```python
from build123d import *

# Parameters (mm, degrees)
F1_DEPTH       = 15
F2_R           = 2
F4_DEPTH       = 4.5
F6_DEPTH       = 4.5
F7_R           = 2
F8_SIZE        = 1
F10_DEPTH      = 2
F10_DEPTH_BACK = 8
F12_DEPTH      = 5
F14_DEPTH      = 1
F15_R          = 10
F16_R          = 3
F17_R          = 2
F18_T1_DEPTH   = 27


# Not quite as in the source:
# - a fillet or chamfer that OpenCascade refuses, or shapes differently, is made with other operations: its cross-section is extruded or revolved along the edge and cut away or added


with BuildPart() as f1:
    # F0 (on Top) → F1 (new body)
    with BuildSketch(Plane.XY):
        Polygon((-8.0448907178, 7.5019819607), (0, 0), (15.0350819326, 5.4723222932), (25.8464898551, 56.3359975314), (19.5579639798, 92), (-3.4420360202, 92), (-8.030647511, 85.4467836457), (-6.4537553867, 81.7707244475), (-13.8947211419, 53.7415962301), (-16.7171564284, 43.1098579407), (-19.7961767409, 31.5115979887), (-9.299232277, 19.4362447051), align=None)
        with BuildLine():
            ThreePointArc((-13.8947211419, 53.7415962301), (-18.2055037731, 49.1954821635), (-16.7171564284, 43.1098579407))
            Line((-16.7171564284, 43.1098579407), (-13.8947211419, 53.7415962301))
        make_face()
    extrude(amount=F1_DEPTH)

    # F2
    f2_edges = [f1.edges().sort_by_distance(p)[0] for p in [
        (-3.442036, 92, 7.5),
        (19.557964, 92, 7.5),
        (-8.030648, 85.446784, 7.5),
        (-6.453755, 81.770724, 7.5),
        (25.84649, 56.335998, 7.5),
        (15.035082, 5.472322, 7.5),
        (-19.796177, 31.511598, 7.5),
        (-8.044891, 7.501982, 7.5),
        (0, 0, 7.5),
    ]]
    fillet(f2_edges, radius=F2_R)

    # F3 (on face) → F4 (cut)
    with BuildSketch(Plane.XY.offset(15)):
        with BuildLine():
            Line((-19.1004557272, 30.7112625143), (-9.299232277, 19.4362447051))
            Line((-9.299232277, 19.4362447051), (-9.9431083431, 25.5623162612))
            ThreePointArc((-9.9431083431, 25.5623162612), (-4.1654007718, 41.7730592838), (-4.2262892289, 58.9825446545))
            Line((-4.2262892289, 58.9825446545), (0.2837840411, 62.9397203012))
            Line((0.2837840411, 62.9397203012), (-1.9921549357, 80.795254507))
            Line((-1.9921549357, 80.795254507), (-6.7258938789, 82.4051351292))
            ThreePointArc((-6.7258938789, 82.4051351292), (-6.5692308005, 81.7622951194), (-6.6308801526, 81.103519015))
            Line((-6.6308801526, 81.103519015), (-13.8947211419, 53.7415962301))
            ThreePointArc((-13.8947211419, 53.7415962301), (-18.2055037731, 49.1954821635), (-16.7171564284, 43.1098579407))
            Line((-16.7171564284, 43.1098579407), (-19.5240798921, 32.5365506243))
            ThreePointArc((-19.5240798921, 32.5365506243), (-19.539255282, 31.5712259114), (-19.1004557272, 30.7112625143))
        make_face()
    extrude(amount=-F4_DEPTH, mode=Mode.SUBTRACT)

    # F5 (on face) → F6 (cut)
    with BuildSketch(Plane(origin=(0, 0, 0), x_dir=(1, 0, 0), z_dir=(0, 0, -1))):
        with BuildLine():
            ThreePointArc((-6.6308801526, -81.103519015), (-6.5692308005, -81.7622951194), (-6.7258938789, -82.4051351292))
            Line((-6.7258938789, -82.4051351292), (-2.0079532375, -80.7495276563))
            Line((-2.0079532375, -80.7495276563), (0.2709017201, -62.8943653752))
            Line((0.2709017201, -62.8943653752), (-4.2385252382, -58.9364532352))
            ThreePointArc((-4.2385252382, -58.9364532352), (-4.1797341848, -41.7514896804), (-9.9430388376, -25.5616549609))
            Line((-9.9430388376, -25.5616549609), (-9.299232277, -19.4362447051))
            Line((-9.299232277, -19.4362447051), (-19.1004557272, -30.7112625143))
            ThreePointArc((-19.1004557272, -30.7112625143), (-19.539255282, -31.5712259114), (-19.5240798921, -32.5365506243))
            Line((-19.5240798921, -32.5365506243), (-16.7171564284, -43.1098579407))
            ThreePointArc((-16.7171564284, -43.1098579407), (-18.2055037731, -49.1954821635), (-13.8947211419, -53.7415962301))
            Line((-13.8947211419, -53.7415962301), (-6.6308801526, -81.103519015))
        make_face()
    extrude(amount=-F6_DEPTH, mode=Mode.SUBTRACT)

    # F7
    f7_edges = [f1.edges().sort_by_distance(p)[0] for p in [
        (-9.943108, 25.562316, 12.75),
        (-9.943039, 25.561655, 2.25),
        (-4.226289, 58.982545, 12.75),
        (0.283784, 62.93972, 12.75),
        (-4.238525, 58.936453, 2.25),
        (0.270902, 62.894365, 2.25),
        (-1.992155, 80.795255, 12.75),
        (-2.007953, 80.749528, 2.25),
        (-6.725894, 82.405135, 7.5),
        (-6.725894, 82.405135, 2.25),
        (-6.725894, 82.405135, 12.75),
    ]]
    fillet(f7_edges, radius=F7_R)

    # F8
    f8_edges = [f1.edges().sort_by_distance(p)[0] for p in [
        (-7.334289, 83.82343, 15),
        (-6.597337, 82.544049, 15),
        (-7.743054, 85.417108, 15),
        (-4.528565, 81.657853, 15),
        (-5.715563, 88.753067, 15),
        (-2.269238, 80.568943, 15),
        (-3.324399, 91.774022, 15),
        (-0.842477, 71.775634, 15),
        (7.739431, 92, 15),
        (0.035819, 63.033597, 15),
        (19.16534, 91.532089, 15),
        (-1.952405, 60.977669, 15),
        (22.814181, 73.533074, 15),
        (-3.950317, 58.895605, 15),
        (25.809062, 56.336651, 15),
        (-4.205609, 41.541288, 15),
        (20.515619, 31.256223, 15),
        (-9.848308, 25.536603, 15),
        (14.818701, 5.66042, 15),
        (-8.999956, 16.588822, 15),
        (7.572505, 2.756166, 15),
        (-7.923879, 7.562316, 15),
        (0.068913, 0.338716, 15),
        (-4.197178, 3.913931, 15),
        (-7.332009, 83.818114, 0),
        (-6.599862, 82.540006, 0),
        (-7.743054, 85.417108, 0),
        (-4.534925, 81.636286, 0),
        (-5.715563, 88.753067, 0),
        (-2.280519, 80.529059, 0),
        (-3.324399, 91.774022, 0),
        (-0.857666, 71.736857, 0),
        (7.739431, 92, 0),
        (0.022922, 62.988201, 0),
        (19.16534, 91.532089, 0),
        (-1.965224, 60.931724, 0),
        (22.814181, 73.533074, 0),
        (-3.962878, 58.849592, 0),
        (25.809062, 56.336651, 0),
        (-4.219912, 41.519712, 0),
        (20.515619, 31.256223, 0),
        (-9.848432, 25.536019, 0),
        (14.818701, 5.66042, 0),
        (-8.999957, 16.588832, 0),
        (7.572505, 2.756166, 0),
        (-7.923879, 7.562316, 0),
        (0.068913, 0.338716, 0),
        (-4.197178, 3.913931, 0),
    ]]
    chamfer(f8_edges, length=F8_SIZE)

    # F9 (on face) → F10 (join, two sides)
    with BuildSketch(Plane.XY.offset(10.5)) as f10_sk:
        Polygon((-9.2121738851, 71.3801288833), (-11.82835392, 61.5253266909), (-8.928788932, 60.7555716127), (-7.6458638018, 65.5881799261), (-5.5294538555, 67.7143993266), align=None)
    extrude(amount=F10_DEPTH)
    extrude(f10_sk.sketch, amount=-F10_DEPTH_BACK)

    # F11 (on face) → F12 (join)
    with BuildSketch(Plane(origin=(0, 0, 0), x_dir=(1, 0, 0), z_dir=(0, 0, -1))):
        Polygon((5.5166269788, -69.1855618273), (14.7091602962, -76.8990131435), (15.3519479059, -76.1329687004), (6.1594145885, -68.4195173842), align=None)
    extrude(amount=F12_DEPTH)

    # F13 (on face) → F14 (join)
    with BuildSketch(Plane(origin=(0, 0, -5), x_dir=(1, 0, 0), z_dir=(0, 0, -1))):
        Polygon((6.1594145885, -68.4195173842), (15.3519479059, -76.1329687004), (18.3099562872, -59.3572695449), (9.9443103961, -20), (4.371628125, -21.1845101828), (8.5288556293, -61.3816455007), align=None)
        Polygon((14.7091602962, -76.8990131435), (15.3519479059, -76.1329687004), (6.1594145885, -68.4195173842), (5.5166269788, -69.1855618273), align=None)
    extrude(amount=-F14_DEPTH)

    # F15
    f15_edges = [f1.edges().sort_by_distance(p)[0] for p in [
        (18.309956, 59.35727, -4.5),
        (8.528856, 61.381646, -4.5),
    ]]
    fillet(f15_edges, radius=F15_R)

    # F16
    f16_edges = [f1.edges().sort_by_distance(p)[0] for p in [
        (4.371628, 21.18451, -4.5),
        (9.94431, 20, -4.5),
    ]]
    fillet(f16_edges, radius=F16_R)

    # F17
    f17_edges = [f1.edges().sort_by_distance(p)[0] for p in [
        (10.755681, 72.276243, -4),
    ]]
    fillet(f17_edges, radius=F17_R)

    # F18: fillet of radius 3 on 1 edges, made by hand

    # F18_s2 → F18_t1 (cut)
    with BuildSketch(Plane(origin=(31.5591951189, 26.4813089845, 0), x_dir=(0, 0, 1), z_dir=(0.7660444431, 0.6427876097, 0))):
        with BuildLine():
            ThreePointArc((-5, -46.4531957126), (-4.1213203436, -48.5745160562), (-2, -49.4531957126))
            Line((-2, -49.4531957126), (-5, -49.4531957126))
            Line((-5, -49.4531957126), (-5, -46.4531957126))
        make_face()
    extrude(amount=F18_T1_DEPTH, mode=Mode.SUBTRACT)


solid = f1.part
```
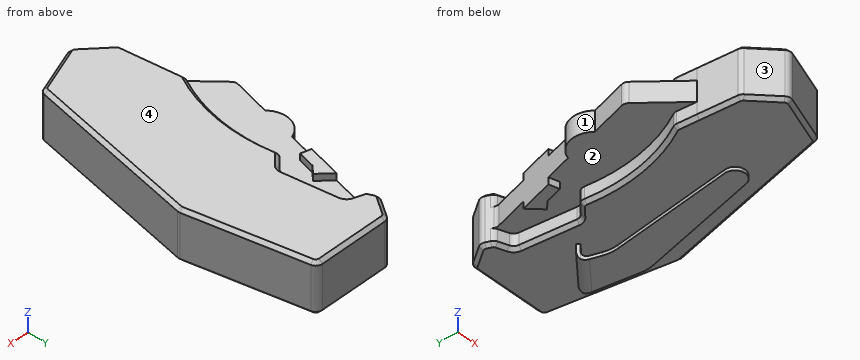
The model under review builds one solid part; all positions refer to its coordinate system, in mm. Face numbers are marked on the shaded views. Give positions to 0.01 mm unless a question says otherwise; leave off trailing zeros. Order: outer loops, then holes, each group sorted by start corner. A loop starts at its lowest first (then second) coordinate and runs counter-clockwise, first axis right, second up. Notation, with made-up numbers: (73.25, -15.5) - (84.25, -15.5) arc R28 ccw to (84.25, 14.5) - close; hole circle Ø2 at (-37.5, 5.25). An arc over 180 degrees is marked (long way). Use CSV: the item, a comma, the result in double quotes. Start each with the question number.
Q1. We need section B-B, the plane x = 21. Write out the cut boundary in (y, z), and give its area (3 significant figures).
Q2. The part is to be moulded in two halves that separate along Y. For the marked faces 1, 2, 3 and 4, say which applies: +Y half, -Y half, draft (parallel to the pull), parting line (faces both ways), or undercut.
Q3. To check wall thickness, follow line 1 along Z through (x, y) = (6.5, 33.5); line 2 along Z through (x, y) = (-8, 68); line 3 along Z through (x, y) = (-6, 84). State the ranges of each line that lie inside material, in increasing order. Write a range as [from, to].
Q4. Clearance check with flat-ended pins moving along their axes: pin 1 Ø1 at (y, z) = (33.5, 12) entering from +X; pin 2 Ø6 at (y, z) = (35, 10) entering from +X; pin 3 Ø10 at (x, z) = (-9.5, 3) entering from +Y. State where each tip first meets the part, or that it passes through.
Q5. We need section A-A, the plane z = 7. Write out the cut boundary in (x, y), and give its area (3 significant figures).
Outcome:
1,outline,"(33.54, 1) - (38.34, 0) - (78.06, 0) - (83.82, 1) - (83.82, 14) - (78.06, 15) - (38.34, 15) - (33.54, 14) - close"
1,area,"744 mm^2"
2,face 1,"undercut"
2,face 2,"undercut"
2,face 3,"-Y half"
2,face 4,"draft"
3,line 1,"z = [-5, -4], [0, 15]"
3,line 2,"z = [2.5, 12.5]"
3,line 3,"z = [0, 15]"
4,pin 1,"stops at x = 21.1"
4,pin 2,"stops at x = 21.95"
4,pin 3,"stops at y = 90.49"
5,outline,"(-19.52, 32.54) arc R2 ccw to (-19.1, 30.71) - (-9.3, 19.44) - (-8.12, 8.25) arc R2 ccw to (-7.5, 6.99) - (-0.9, 0.84) arc R2 ccw to (1.15, 0.42) - (13.99, 5.09) arc R2 ccw to (15.27, 6.56) - (25.77, 55.96) arc R2 ccw to (25.78, 56.72) - (19.85, 90.35) arc R2 ccw to (17.88, 92) - (-2.4, 92) arc R2 ccw to (-4.04, 91.15) - (-7.39, 86.36) arc R2 ccw to (-7.59, 84.42) - (-6.73, 82.41) arc R2 cw to (-6.63, 81.1) - (-13.89, 53.74) arc R6.54 ccw to (-16.72, 43.11) - close"
5,area,"2,950 mm^2"
